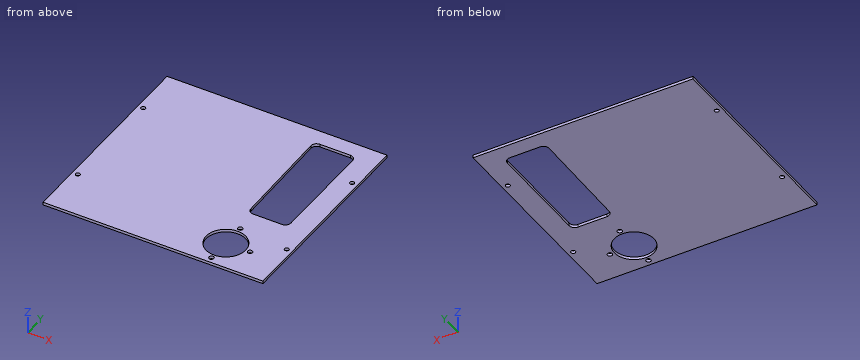
```python
from build123d import *

# Parameters (mm, degrees)
SKETCH1_W           = 100
SKETCH1_H           = 94.92
BOSS_EXTRUDE1_DEPTH = 1.27
SKETCH14_R          = 9
SKETCH14_R_2        = 8
SKETCH14_R_3        = 6
SKETCH14_R_4        = 1.1
CUT_EXTRUDE8_DEPTH  = 5
SKETCH15_R          = 1
CUT_EXTRUDE9_DEPTH  = 10
CUT_EXTRUDE11_DEPTH = 2.54


with BuildPart() as part:
    # Sketch1 → Boss-Extrude1 (new body)
    with BuildSketch(Plane.XY):
        with Locations((50, 48.73)):
            Rectangle(SKETCH1_W, SKETCH1_H)
    extrude(amount=BOSS_EXTRUDE1_DEPTH)

    # Sketch14 → Cut-Extrude8 (cut)
    with BuildSketch(Plane(origin=(0, 0, 0), x_dir=(-1, 0, 0), z_dir=(0, 0, -1))):
        with Locations((-75, 15)):
            Circle(SKETCH14_R)
        with Locations((-75, 15)):
            Circle(SKETCH14_R_2, mode=Mode.SUBTRACT)
        with Locations((-75, 15)):
            Circle(SKETCH14_R_2)
        with Locations((-75, 15)):
            Circle(SKETCH14_R_3, mode=Mode.SUBTRACT)
        with Locations((-75, 15)):
            Circle(SKETCH14_R_3)
        with Locations((-75, 26)):
            Circle(SKETCH14_R_4)
        with Locations((-86, 15)):
            Circle(SKETCH14_R_4)
        with Locations((-75, 4)):
            Circle(SKETCH14_R_4)
    extrude(amount=-CUT_EXTRUDE8_DEPTH, mode=Mode.SUBTRACT)

    # Sketch15 → Cut-Extrude9 (cut)
    with BuildSketch(Plane(origin=(0, 0, 0), x_dir=(-1, 0, 0), z_dir=(0, 0, -1))):
        with Locations(Location((-2.5, 73.73, 0), (0, 0, 180))):
            Circle(SKETCH15_R)
        with Locations(Location((-2.5, 23.73, 0), (0, 0, 180))):
            Circle(SKETCH15_R)
        with Locations((-97.5, 23.73)):
            Circle(SKETCH15_R)
        with Locations((-97.5, 73.73)):
            Circle(SKETCH15_R)
    extrude(amount=-CUT_EXTRUDE9_DEPTH, mode=Mode.SUBTRACT)

    # Sketch18 → Cut-Extrude11 (cut)
    with BuildSketch(Plane.XY.offset(1.27)):
        with BuildLine():
            Line((87.669088652, 88.855847161), (73.816841533, 88.855847161))
            ThreePointArc((73.816841533, 88.855847161), (72.007429626, 88.098437566), (71.277124758, 86.277916888))
            Line((71.277124758, 86.277916888), (71.981132893, 39.139282942))
            ThreePointArc((71.981132893, 39.139282942), (72.738259262, 37.367801309), (74.520849667, 36.637213215))
            Line((74.520849667, 36.637213215), (87.669088652, 36.637213215))
            ThreePointArc((87.669088652, 36.637213215), (89.465139876, 37.381161991), (90.209088652, 39.177213215))
            Line((90.209088652, 39.177213215), (90.209088652, 86.315847161))
            ThreePointArc((90.209088652, 86.315847161), (89.465139876, 88.111898385), (87.669088652, 88.855847161))
        make_face()
    extrude(amount=-CUT_EXTRUDE11_DEPTH, mode=Mode.SUBTRACT)


solid = part.part
```
Input: part model. Units: mm. Frame: model coordinates. Coordinates: 2 decimals unless noted, no trailing zeros. Loops run counter-clockwise (first coordinate to the right, second up) from the corner with the lowest first, then second, coordinate; pieces in that order, holes last. Notation, with made-up numbers: (58.25, -11) -> (107.25, -11) arc R25 ccw to (107.25, 9) -> close; hole circle Ø3 at (51, -36). An arc over 180 degrees is marked (long way). Use a Markdown table: item, result.
1) Cut plane B-B (y = 60). Return the cut outline in (x, z), then the cut area to 3 significant figures.
Results found:
| item | result |
|---|---|
| outline | (0, 0) -> (71.67, 0) -> (71.67, 1.27) -> (0, 1.27) -> close; (90.21, 0) -> (100, 0) -> (100, 1.27) -> (90.21, 1.27) -> close |
| area | 103 mm2 |
2) Contact query for flat-ended pins moving along their axis: pin 1 (5 mm diameter, centred on x = 70, y = 55.5, fed in from -Z); pin 2 (1.8 mm diameter, centred on x = 86, y = 15, fed in from -Z). Output: stop coordinate, or through.
Results found:
| item | result |
|---|---|
| pin 1 | stops at z = 0 |
| pin 2 | passes through |
3) Material intervals for line 1 along Y through (x, z) = (2.5, 0.8); line 2 along Y through (x, z) = (75, 0.5); line 3 along Y through (x, z) = (87.5, 0.7), sorted ascending. Write a range as from..to.
Results found:
| item | result |
|---|---|
| line 1 | y = 1.27..22.73, 24.73..72.73, 74.73..96.19 |
| line 2 | y = 1.27..2.9, 5.1..6, 24..24.9, 27.1..36.64, 88.86..96.19 |
| line 3 | y = 1.27..36.64, 88.86..96.19 |
4) Cut plane C-C (y = 46). Return the cut outline in (x, z), then the cut area to 3 significant figures.
Results found:
| item | result |
|---|---|
| outline | (0, 0) -> (71.88, 0) -> (71.88, 1.27) -> (0, 1.27) -> close; (90.21, 0) -> (100, 0) -> (100, 1.27) -> (90.21, 1.27) -> close |
| area | 104 mm2 |
5) Cut plane A-A (z = 0.8). Give the number of separate pieces and of enclosed holes in the cut face, then the cut area to 3 significant figures.
Results found:
| item | result |
|---|---|
| separate pieces | 1 |
| enclosed holes | 9 |
| area | 8,250 mm2 |
